```python
from build123d import *

# Parameters (mm, degrees)
ESQUISSE1_W             = 150
ESQUISSE1_H             = 125
BOSS_EXTRU_3_DEPTH      = 2
BOSS_EXTRU_4_DEPTH      = 51
BOSS_EXTRU_6_DEPTH      = 47
ESQUISSE1_9_R           = 3.2
ESQUISSE1_9_R_2         = 1.6
BOSS_EXTRU_7_DEPTH      = 5
ESQUISSE3_W             = 18
ESQUISSE3_H             = 16
ESQUISSE3_W_2           = 10
ESQUISSE3_H_2           = 7
ENL_V_MAT_EXTRU_1_DEPTH = 15
ESQUISSE4_W             = 5
ESQUISSE4_H             = 11
ENL_V_MAT_EXTRU_2_DEPTH = 15
ESQUISSE1_12_W          = 8
ESQUISSE1_12_H          = 12
ESQUISSE1_12_R          = 1.6
BOSS_EXTRU_8_DEPTH      = 51
CONG_5_R                = 4


with BuildPart() as part:
    # Esquisse1 → Boss.-Extru.3 (new body)
    with BuildSketch(Plane.XY):
        with Locations((80, 67.5)):
            Rectangle(ESQUISSE1_W, ESQUISSE1_H)
    extrude(amount=BOSS_EXTRU_3_DEPTH)

    # Esquisse1_6 → Boss.-Extru.4 (add)
    with BuildSketch(Plane.XY):
        with BuildLine():
            ThreePointArc((2.5, 5), (3.232233047, 3.232233047), (5, 2.5))
            Line((5, 2.5), (155, 2.5))
            ThreePointArc((155, 2.5), (156.767766953, 3.232233047), (157.5, 5))
            Line((157.5, 5), (157.5, 130))
            ThreePointArc((157.5, 130), (156.767766953, 131.767766953), (155, 132.5))
            Line((155, 132.5), (5, 132.5))
            ThreePointArc((5, 132.5), (3.232233047, 131.767766953), (2.5, 130))
            Line((2.5, 130), (2.5, 5))
        make_face()
        Polygon((147, 5), (5, 5), (5, 118), (5, 130), (13, 130), (147, 130), (155, 130), (155, 118), (155, 17), (155, 5), align=None, mode=Mode.SUBTRACT)
    extrude(amount=BOSS_EXTRU_4_DEPTH)

    # Esquisse1_8 → Boss.-Extru.6 (add)
    # profile 1 of 5: a face of its own
    with BuildSketch(Plane.XY):
        with BuildLine():
            ThreePointArc((0, 2.5), (0.732233047, 0.732233047), (2.5, 0))
            Line((2.5, 0), (157.5, 0))
            ThreePointArc((157.5, 0), (159.267766953, 0.732233047), (160, 2.5))
            Line((160, 2.5), (160, 132.5))
            ThreePointArc((160, 132.5), (159.267766953, 134.267766953), (157.5, 135))
            Line((157.5, 135), (2.5, 135))
            ThreePointArc((2.5, 135), (0.732233047, 134.267766953), (0, 132.5))
            Line((0, 132.5), (0, 2.5))
        make_face()
        Polygon((5, 2.5), (2.5, 2.5), (2.5, 5), (2.5, 130), (2.5, 132.5), (5, 132.5), (155, 132.5), (157.5, 132.5), (157.5, 130), (157.5, 5), (157.5, 2.5), (155, 2.5), align=None, mode=Mode.SUBTRACT)
    # profile 2 of 5: a face of its own
    with BuildSketch(Plane.XY):
        with BuildLine():
            Line((2.5, 132.5), (2.5, 130))
            ThreePointArc((2.5, 130), (3.232233047, 131.767766953), (5, 132.5))
            Line((5, 132.5), (2.5, 132.5))
        make_face()
    # profile 3 of 5: a face of its own
    with BuildSketch(Plane.XY):
        with BuildLine():
            ThreePointArc((155, 132.5), (156.767766953, 131.767766953), (157.5, 130))
            Line((157.5, 130), (157.5, 132.5))
            Line((157.5, 132.5), (155, 132.5))
        make_face()
    # profile 4 of 5: a face of its own
    with BuildSketch(Plane.XY):
        with BuildLine():
            ThreePointArc((157.5, 5), (156.767766953, 3.232233047), (155, 2.5))
            Line((155, 2.5), (157.5, 2.5))
            Line((157.5, 2.5), (157.5, 5))
        make_face()
    # profile 5 of 5: a face of its own
    with BuildSketch(Plane.XY):
        with BuildLine():
            Line((2.5, 5), (2.5, 2.5))
            Line((2.5, 2.5), (5, 2.5))
            ThreePointArc((5, 2.5), (3.232233047, 3.232233047), (2.5, 5))
        make_face()
    extrude(amount=BOSS_EXTRU_6_DEPTH)

    # Esquisse1_9 → Boss.-Extru.7 (add)
    # profile 1 of 4: a face of its own
    with BuildSketch(Plane.XY):
        with Locations((142, 112)):
            Circle(ESQUISSE1_9_R)
        with Locations((142, 112)):
            Circle(ESQUISSE1_9_R_2, mode=Mode.SUBTRACT)
    # profile 2 of 4: a face of its own
    with BuildSketch(Plane.XY):
        with Locations((10, 112)):
            Circle(ESQUISSE1_9_R)
        with Locations((10, 112)):
            Circle(ESQUISSE1_9_R_2, mode=Mode.SUBTRACT)
    # profile 3 of 4: a face of its own
    with BuildSketch(Plane.XY):
        with Locations((10, 10)):
            Circle(ESQUISSE1_9_R)
        with Locations((10, 10)):
            Circle(ESQUISSE1_9_R_2, mode=Mode.SUBTRACT)
    # profile 4 of 4: a face of its own
    with BuildSketch(Plane.XY):
        with Locations((142, 10)):
            Circle(ESQUISSE1_9_R)
        with Locations((142, 10)):
            Circle(ESQUISSE1_9_R_2, mode=Mode.SUBTRACT)
    extrude(amount=BOSS_EXTRU_7_DEPTH)

    # Esquisse3 → Enl_v. mat.-Extru.1 (cut)
    with BuildSketch(Plane.XZ):
        with Locations((117, 14)):
            Rectangle(ESQUISSE3_W, ESQUISSE3_H)
        with Locations((40.5, 9.5)):
            Rectangle(ESQUISSE3_W_2, ESQUISSE3_H_2)
    extrude(amount=-ENL_V_MAT_EXTRU_1_DEPTH, mode=Mode.SUBTRACT)

    # Esquisse4 → Enl_v. mat.-Extru.2 (cut)
    with BuildSketch(Plane.ZY):
        with Locations((8.5, 19)):
            Rectangle(ESQUISSE4_W, ESQUISSE4_H)
    extrude(amount=-ENL_V_MAT_EXTRU_2_DEPTH, mode=Mode.SUBTRACT)

    # Esquisse1_12 → Boss.-Extru.8 (add)
    # profile 1 of 3: a face of its own
    with BuildSketch(Plane.XY):
        with Locations((151, 11)):
            Rectangle(ESQUISSE1_12_W, ESQUISSE1_12_H)
        with Locations((151, 11)):
            Circle(ESQUISSE1_12_R, mode=Mode.SUBTRACT)
    # profile 2 of 3: a face of its own
    with BuildSketch(Plane.XY):
        with Locations((9, 124)):
            Rectangle(ESQUISSE1_12_W, ESQUISSE1_12_H)
        with Locations((9, 124)):
            Circle(ESQUISSE1_12_R, mode=Mode.SUBTRACT)
    # profile 3 of 3: a face of its own
    with BuildSketch(Plane.XY):
        with Locations((151, 124)):
            Rectangle(ESQUISSE1_12_W, ESQUISSE1_12_H)
        with Locations((151, 124)):
            Circle(ESQUISSE1_12_R, mode=Mode.SUBTRACT)
    extrude(amount=BOSS_EXTRU_8_DEPTH)

    # Cong_5
    cong_5_edges = [part.edges().sort_by_distance(p)[0] for p in [
        (147, 118, 26.5),
        (147, 17, 26.5),
        (13, 118, 26.5),
    ]]
    fillet(cong_5_edges, radius=CONG_5_R)


solid = part.part
```
Check sheet for the modelled part. Datum: model origin and axes. Units: mm. A direction names the side the tool comes from. Round coordinates to 2 decimals unless told otherwise and drop trailing zeros. Order: outer loops, then holes, each group sorted by start corner. A loop starts at its lowest first (then second) coordinate and runs counter-clockwise, first axis right, second up. Notation, with made-up numbers: (16.5, -8) -> (73.5, -8) arc R24 cw to (73.5, 30) -> close; hole circle Ø6 at (56.5, 63). An arc over 180 degrees is marked (long way). One line per item, written item: value. Start each with the question number.
Q1. Cross-section at C-C (z = 16). Record the boundary of the cut face in (x, y).
Q2. Gauge pin test, flat ends, axial feed: pin 1 Ø3 at (x, y) = (142, 10) entering from +Z; pin 2 Ø4 at (x, z) = (119.5, 10) entering from -Y. Record the tip position at first contact, or that the pin passes through.
Q3. Cross-section at A-A (z = 32). Record the boundary of the cut face in (x, y), and give its area (3 significant figures).
Q4. Thickness scan on line 1 (X direction, y = 112, z = 4.2); line 2 (Y direction, x = 142, z = 2.9); line 3 (X direction, y = 92.5, z = 38.5). Record the ranges inside material, lowest first.
Q5. Set-up check for faces 4 (the face through (11.4, 110.6, 5)), 5 (the face through (2, 24.5, 8)), 6 (the face through (126, 2, 14)): record each of +Z, -Z, +X, -X, +Y, -Y from which the full face is reachable in a straight line by a thin tool's end or side.
Q6. Cross-section at D-D (y = 105). Record the boundary of the cut face in (x, z).
Q7. Cross-section at B-B (x = 112). Record the boundary of the cut face in (y, z), and give its area (3 significant figures).
Q8. Mould release check, pull along Y, two halves, no side actions. Record for faces 1 (the face through (79, 68, 2)), 2 (the face through (81, 132.5, 49)), 3 (the face through (117, 2, 6)): pulls with the +Y half, pulls with the -Y half, needs draft (parallel to the pull), parting line crosses it, or undercut.
Completed:
1. outline: (0, 2.5) arc R2.5 ccw to (2.5, 0) -> (108, 0) -> (108, 5) -> (5, 5) -> (5, 118) -> (9, 118) arc R4 ccw to (13, 122) -> (13, 130) -> (147, 130) -> (147, 122) arc R4 ccw to (151, 118) -> (155, 118) -> (155, 17) -> (151, 17) arc R4 ccw to (147, 13) -> (147, 5) -> (126, 5) -> (126, 0) -> (157.5, 0) arc R2.5 ccw to (160, 2.5) -> (160, 132.5) arc R2.5 ccw to (157.5, 135) -> (2.5, 135) arc R2.5 ccw to (0, 132.5) -> close; hole circle Ø3.2 at (9, 124); hole circle Ø3.2 at (151, 11); hole circle Ø3.2 at (151, 124)
2. pin 1: stops at z = 2
2. pin 2: stops at y = 130
3. outline: (0, 2.5) arc R2.5 ccw to (2.5, 0) -> (157.5, 0) arc R2.5 ccw to (160, 2.5) -> (160, 132.5) arc R2.5 ccw to (157.5, 135) -> (2.5, 135) arc R2.5 ccw to (0, 132.5) -> close; hole (5, 5) -> (147, 5) -> (147, 13) arc R4 cw to (151, 17) -> (155, 17) -> (155, 118) -> (151, 118) arc R4 cw to (147, 122) -> (147, 130) -> (13, 130) -> (13, 122) arc R4 cw to (9, 118) -> (5, 118) -> close; hole circle Ø3.2 at (9, 124); hole circle Ø3.2 at (151, 11); hole circle Ø3.2 at (151, 124)
3. area: 3,100 mm²
4. line 1: x = 0 to 5, 6.8 to 8.4, 11.6 to 13.2, 138.8 to 140.4, 143.6 to 145.2, 155 to 160
4. line 2: y = 0 to 5, 6.8 to 8.4, 11.6 to 13.2, 108.8 to 110.4, 113.6 to 115.2, 130 to 135
4. line 3: x = 0 to 5, 155 to 160
5. face 4: +Z
5. face 5: -X
5. face 6: -Y
6. outline: (0, 0) -> (160, 0) -> (160, 47) -> (157.5, 47) -> (157.5, 51) -> (155, 51) -> (155, 2) -> (5, 2) -> (5, 51) -> (2.5, 51) -> (2.5, 47) -> (0, 47) -> close
7. outline: (0, 0) -> (135, 0) -> (135, 47) -> (132.5, 47) -> (132.5, 51) -> (130, 51) -> (130, 2) -> (5, 2) -> (5, 6) -> (0, 6) -> close; (0, 22) -> (5, 22) -> (5, 51) -> (2.5, 51) -> (2.5, 47) -> (0, 47) -> close
7. area: 660 mm²
8. face 1: undercut
8. face 2: pulls with the +Y half
8. face 3: needs draft
